from build123d import *

# Parameters (mm, degrees)
SKETCH_1_W      = 70
SKETCH_1_H      = 85
SKETCH_1_R      = 1.5
SKETCH_1_R_2    = 1.25
EXTRUDE_1_DEPTH = 2
FILLET_1_R      = 2


with BuildPart() as part:
    # 草图1 → 凸台-拉伸1 (new body)
    with BuildSketch(Plane.XY):
        Rectangle(SKETCH_1_W, SKETCH_1_H)
        with Locations((-20, 15)):
            Circle(SKETCH_1_R, mode=Mode.SUBTRACT)
        with Locations((20, 15)):
            Circle(SKETCH_1_R, mode=Mode.SUBTRACT)
        with Locations((-20, -15)):
            Circle(SKETCH_1_R, mode=Mode.SUBTRACT)
        with Locations((20, -15)):
            Circle(SKETCH_1_R, mode=Mode.SUBTRACT)
        with Locations((10.1, 10.1)):
            Circle(SKETCH_1_R_2, mode=Mode.SUBTRACT)
        with Locations((-10.1, -10.1)):
            Circle(SKETCH_1_R_2, mode=Mode.SUBTRACT)
        Circle(SKETCH_1_R_2, mode=Mode.SUBTRACT)
    extrude(amount=EXTRUDE_1_DEPTH)

    # 圆角1
    fillet_1_edges = [part.edges().sort_by_distance(p)[0] for p in [
        (35, -42.5, 1),
        (-35, -42.5, 1),
        (-35, 42.5, 1),
        (35, 42.5, 1),
    ]]
    fillet(fillet_1_edges, radius=FILLET_1_R)


solid = part.part
The model under review builds one solid part; all positions refer to its coordinate system, in mm. Round coordinates to 2 decimals unless told otherwise and drop trailing zeros. Write each loop counter-clockwise with the first axis right and the second up, starting at its lowest first coordinate (ties: lowest second). Pieces come first, ordered by that corner, then holes. Notation, with made-up numbers: (57.5, 81.5) -> (99.5, 81.5) arc R22 cw to (99.5, 109.5) -> close; hole circle Ø10 at (15.25, 70). An arc over 180 degrees is marked (long way). Answer as a JSON object with one key per item and string values.
1. The part is to be moulded in two halves that separate along Y. For faces 1 (the face through (7, 1, 2)), 2 (the face through (-21.5, 15.07, 0.99)), 3 (the face through (34.4, -41.93, 1.01)), say which applies: pulls with the +Y half, pulls with the -Y half, needs draft (parallel to the pull), parting line crosses it, or undercut.
Results found:
{"face 1": "needs draft", "face 2": "undercut", "face 3": "pulls with the -Y half"}
2. We need section B-B on y = -10.1. State the section outline as (x, z) points, and give its area (3 significant figures).
Results found:
{"outline": "(-35, 0) -> (-11.35, 0) -> (-11.35, 2) -> (-35, 2) -> close; (-8.85, 0) -> (35, 0) -> (35, 2) -> (-8.85, 2) -> close", "area": "135 mm^2"}
3. We need section C-C on y = 15. State the section outline as (x, z) points.
Results found:
{"outline": "(-35, 0) -> (-21.5, 0) -> (-21.5, 2) -> (-35, 2) -> close; (-18.5, 0) -> (18.5, 0) -> (18.5, 2) -> (-18.5, 2) -> close; (21.5, 0) -> (35, 0) -> (35, 2) -> (21.5, 2) -> close"}
4. To check wall thickness, follow line 1 along Y through (x, z) = (-20, 0.55); line 2 along Y through (x, z) = (-19, 0.35); line 3 along Y through (x, z) = (10.1, 1.4). State the ranges of each line that lie inside material, in increasing order.
Results found:
{"line 1": "y = -42.5 to -16.5, -13.5 to 13.5, 16.5 to 42.5", "line 2": "y = -42.5 to -16.12, -13.88 to 13.88, 16.12 to 42.5", "line 3": "y = -42.5 to 8.85, 11.35 to 42.5"}
5. Clearance check with a flat-ended pin moving along its axis: pin 1 (2.5 mm diameter, centred on x = 20, y = -15, fed in from +Z). State where the tip first meets the part, or that it passes through.
Results found:
{"pin 1": "passes through"}
6. We need section A-A on x = 10.1. State the section outline as (y, z) points.
Results found:
{"outline": "(-42.5, 0) -> (8.85, 0) -> (8.85, 2) -> (-42.5, 2) -> close; (11.35, 0) -> (42.5, 0) -> (42.5, 2) -> (11.35, 2) -> close"}
